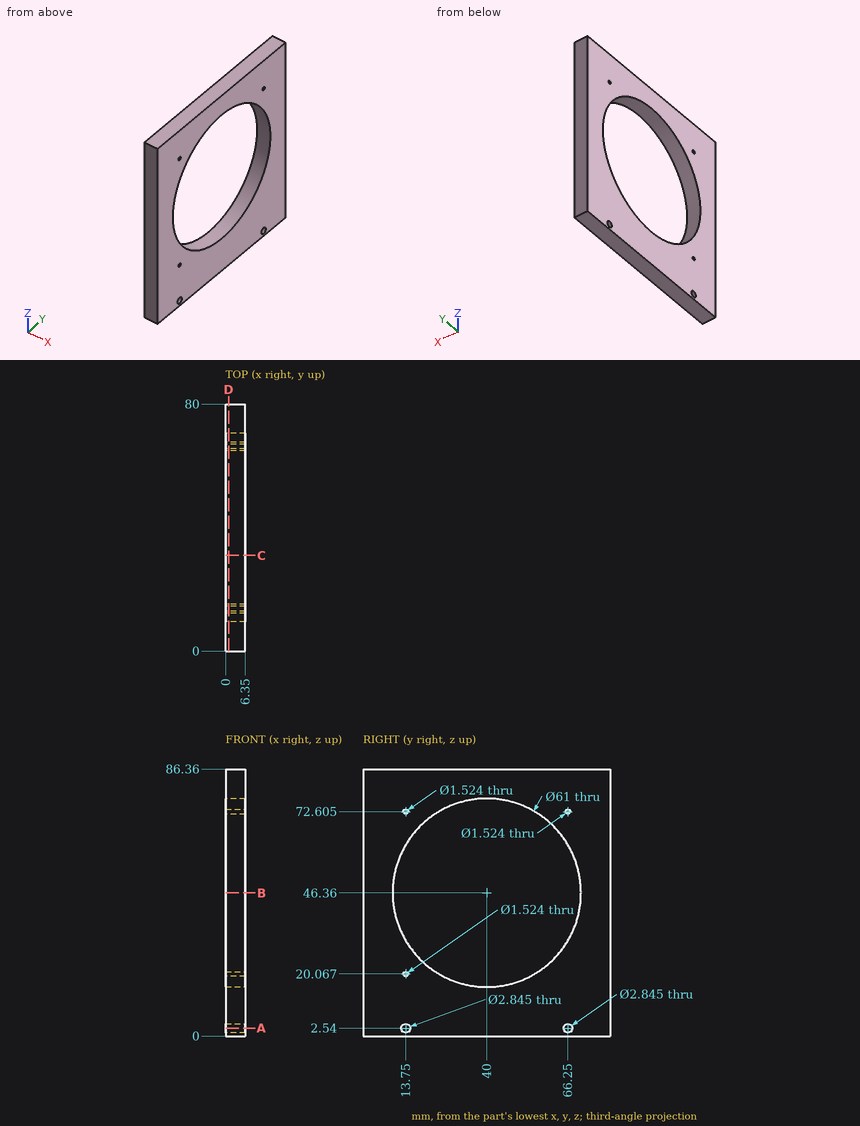
The figure shows three views and two pictorial views of one solid part (mm, origin at its lowest corner). Answer the questions. Round coordinates to 2 decimals unless told otherwise and drop trailing zeros. Write each loop counter-clockwise with the first axis right and the second up, starting at its lowest first coordinate (ties: lowest second). Pieces come first, ordered by that corner, then holes. Notation, with made-up numbers: (-25.75, 72) - (-20.75, 72) arc R17 ccw to (-20.75, 91) - close; hole circle Ø4 at (37.25, 53). An arc over 180 degrees is marked (long way). Answer in a Markdown table with one row per item. Add a question column.
1. A cutting plane is placed at B-B, the plane z = 46.36. Determine the outline of the cut face in (x, y).
2. Given pin 1 (3.5 mm diameter, centred on y = 13.75, z = 2.54, fed in from -X), flat-ended and moving along its own axis, determine where the tip first touches the part or whether it passes through.
3. A cutting plane is placed at D-D, the plane x = 1. Count the separate pieces of the cut face and the enclosed holes in it, and give its area (3 significant figures).
4. Find the intervals of material crossed by line 1 along Z through (x, y) = (1.5, 66.25) (1 decimal); line 2 along Z through (x, y) = (4.5, 15.5) (1 decimal); line 3 along Y through (x, z) = (5, 46.36), in increasing order. Write a range as from..to.
5. A cutting plane is placed at C-C, the plane y = 31. Determine the outline of the cut face in (x, z).
6. A cutting plane is placed at A-A, the plane z = 2.54. Determine the outline of the cut face in (x, y), and give its area (3 significant figures).
Worked out:
| question | item | result |
|---|---|---|
| 1 | outline | (0, 0) - (6.35, 0) - (6.35, 9.5) - (0, 9.5) - close; (0, 70.5) - (6.35, 70.5) - (6.35, 80) - (0, 80) - close |
| 2 | pin 1 | x = 0 |
| 3 | separate pieces | 1 |
| 3 | enclosed holes | 6 |
| 3 | area | 3,970 mm^2 |
| 4 | line 1 | 0..1.1, 4..30.8, 61.9..71.8, 73.4..86.4 |
| 4 | line 2 | 0..28.2, 64.5..86.4 |
| 4 | line 3 | 0..9.5, 70.5..80 |
| 5 | outline | (0, 0) - (6.35, 0) - (6.35, 17.22) - (0, 17.22) - close; (0, 75.5) - (6.35, 75.5) - (6.35, 86.36) - (0, 86.36) - close |
| 6 | outline | (0, 0) - (6.35, 0) - (6.35, 12.33) - (0, 12.33) - close; (0, 15.17) - (6.35, 15.17) - (6.35, 64.83) - (0, 64.83) - close; (0, 67.67) - (6.35, 67.67) - (6.35, 80) - (0, 80) - close |
| 6 | area | 472 mm^2 |
